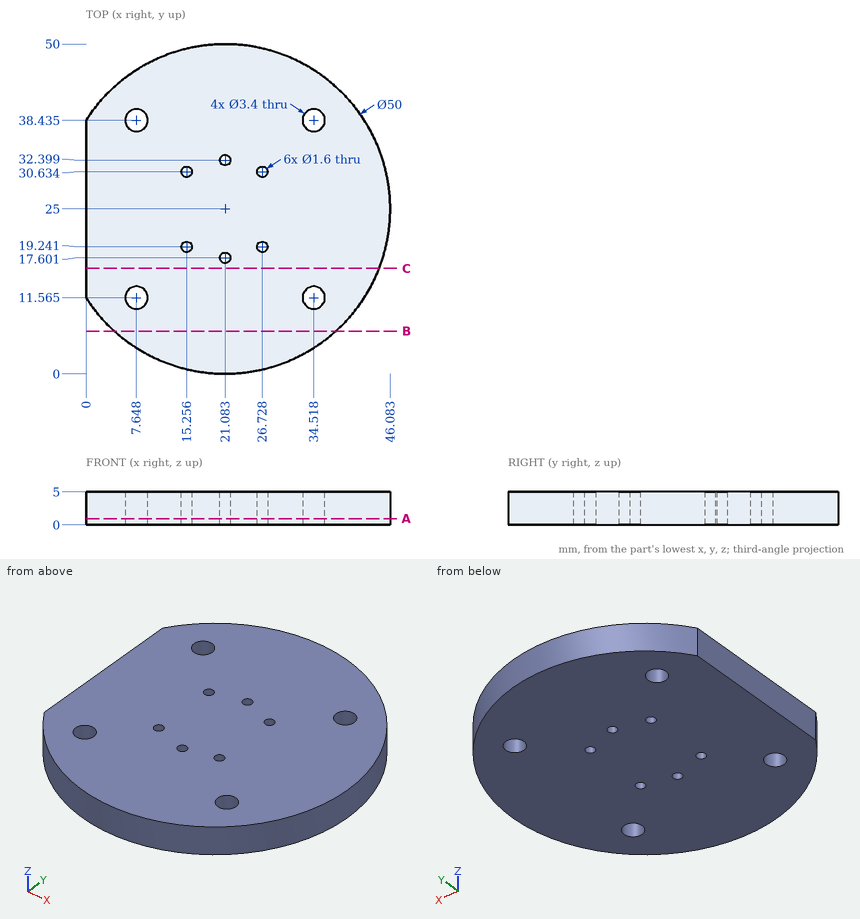
Input: dimensioned drawing with shaded views. Units: mm. Origin: part minimum x, y, z. Round coordinates to 2 decimals unless told otherwise and drop trailing zeros. Order: outer loops, then holes, each group sorted by start corner. A loop starts at its lowest first (then second) coordinate and runs counter-clockwise, first axis right, second up. Notation, with made-up numbers: (22.5, 35) - (70.5, 35) arc R17 cw to (70.5, 68) - close; hole circle Ø10 at (10.5, 20.5). An arc over 180 degrees is marked (long way). Write item = value, one per line. Start each with the question number.
Q1. Cut plane A-A on z = 0.95. Give the number of separate pieces and of enclosed holes in the cut face, and give its area (3 significant figures).
Q2. Cut plane C-C on y = 16. Return the cut outline in (x, z).
Q3. Cut plane B-B on y = 6.5. Return the cut outline in (x, z).
Q4. Pin query (flat end, axial travel): pin 1 (5.5 mm diameter, centred on x = 34.52, y = 11.56, fed in from -Z); pin 2 (3 mm diameter, centred on x = 6, z = 3, fed in from +Y); pin 3 (1 mm diameter, centred on x = 12.5, z = 2, fed in from -Y); pin 4 (1.5 mm diameter, centred on x = 5.5, z = 3, fed in from -Y) (1 decimal). Return the tip coordinate at first contact, or that it passes through.
Q5. Ray query, line 1 (Y direction, x = 35, z = 3.15) (1 decimal); line 2 (Y direction, x = 15.5, z = 2.8) (1 decimal); line 3 (X direction, y = 30.5, z = 1.3) (1 decimal). Return the intervals inside material, ascending. Write a range as from..to.
Outcome:
q1.separate_pieces = 1
q1.enclosed_holes = 10
q1.area = 1,840 mm^2
q2.outline = (0, 0) - (44.41, 0) - (44.41, 5) - (0, 5) - close
q3.outline = (4.27, 0) - (37.9, 0) - (37.9, 5) - (4.27, 5) - close
q4.pin_1 = 0
q4.pin_2 = 45.99
q4.pin_3 = 1.34
q4.pin_4 = 4.9
q5.line_1 = 4.2..9.9, 13.2..36.8, 40.1..45.8
q5.line_2 = 0.6..18.5, 20..29.9, 31.4..49.4
q5.line_3 = 0..14.5, 16..25.9, 27.5..45.5
